from build123d import *

# Parameters (mm, degrees)
SKETCH4_W                               = 180
SKETCH4_H                               = 180
BOSS_EXTRUDE2_DEPTH                     = 10
SKETCH5_R                               = 70
BOSS_EXTRUDE3_DEPTH                     = 80
SKETCH7_R                               = 65
CUT_EXTRUDE1_DEPTH                      = 50
CBORE_FOR_M6_HEX_HEAD_BOLT2_D           = 6.6
CBORE_FOR_M6_HEX_HEAD_BOLT2_CBORE_D     = 14.55
CBORE_FOR_M6_HEX_HEAD_BOLT2_CBORE_DEPTH = 4.38
FILLET1_R                               = 10


with BuildPart() as part:
    # Sketch4 → Boss-Extrude2 (new body)
    with BuildSketch(Plane(origin=(0, 0, 0), x_dir=(1, 0, 0), z_dir=(0, 1, 0))):
        Rectangle(SKETCH4_W, SKETCH4_H)
    extrude(amount=BOSS_EXTRUDE2_DEPTH)

    # Sketch5 → Boss-Extrude3 (add)
    with BuildSketch(Plane(origin=(0, 10, 0), x_dir=(1, 0, 0), z_dir=(0, 1, 0))):
        with Locations(Location((0, 0, 0), (0, 0, 270))):
            Circle(SKETCH5_R)
    extrude(amount=BOSS_EXTRUDE3_DEPTH)

    # Sketch7 → Cut-Extrude1 (cut)
    with BuildSketch(Plane(origin=(0, 90, 0), x_dir=(1, 0, 0), z_dir=(0, 1, 0))):
        with Locations(Location((0, 0, 0), (0, 0, 270))):
            Circle(SKETCH7_R)
    extrude(amount=-CUT_EXTRUDE1_DEPTH, mode=Mode.SUBTRACT)

    # CBORE for M6 Hex Head Bolt2 (through all)
    with Locations(Plane(origin=(0, 10, 0), x_dir=(1, 0, 0), z_dir=(0, 1, 0))):
        with Locations((-75, 75), (75, 75), (75, -75), (-75, -75)):
            CounterBoreHole(CBORE_FOR_M6_HEX_HEAD_BOLT2_D / 2, CBORE_FOR_M6_HEX_HEAD_BOLT2_CBORE_D / 2, CBORE_FOR_M6_HEX_HEAD_BOLT2_CBORE_DEPTH)

    # Fillet1
    fillet1_edges = [part.edges().sort_by_distance(p)[0] for p in [
        (90, 5, 90),
        (-90, 5, 90),
        (-90, 5, -90),
        (90, 5, -90),
    ]]
    fillet(fillet1_edges, radius=FILLET1_R)


solid = part.part
Verification items for the finished model (mm, model axes). A direction names the side the tool comes from. Coordinates: 2 decimals unless noted, no trailing zeros. Order: outer loops, then holes, each group sorted by start corner. A loop starts at its lowest first (then second) coordinate and runs counter-clockwise, first axis right, second up. Notation, with made-up numbers: M 25,83.5 L 50,83.5 A12 cw 50,104.5 Z; hole C 78,4 d11. An arc over 180 degrees is marked long. Return JSON: item names as keys, results as strings.
1) Cross-section at D-D, the plane x = 0. Record the boundary of the cut face in (y, z), and give its area (3 significant figures).
Answer list:
{"outline": "M 0,-90 L 10,-90 L 10,-70 L 90,-70 L 90,-65 L 40,-65 L 40,65 L 90,65 L 90,70 L 10,70 L 10,90 L 0,90 Z", "area": "6,500 mm2"}
2) Cross-section at A-A, the plane z = 75. Record the boundary of the cut face in (x, y) (3 decimals), and give its area (3 significant figures).
Answer list:
{"outline": "M -90,0 L -78.3,0 L -78.3,5.62 L -82.275,5.62 L -82.275,10 L -90,10 Z; M -71.7,0 L 71.7,0 L 71.7,5.62 L 67.725,5.62 L 67.725,10 L -67.725,10 L -67.725,5.62 L -71.7,5.62 Z; M 78.3,0 L 90,0 L 90,10 L 82.275,10 L 82.275,5.62 L 78.3,5.62 Z", "area": "1,600 mm2"}
3) Thickness scan on L1, parallel to X at y = 8, z = 75 (3 decimals); L2, parallel to Z at x = 75, y = 3.85. Record the ranges inside material, lowest first. Write a range as [from, to].
Answer list:
{"L1": "[-90, -82.275], [-67.725, 67.725], [82.275, 90]", "L2": "[-90, -78.3], [-71.7, 71.7], [78.3, 90]"}
4) Access from +Z, -Z, +X, -X, +Y, -Y to the whole of each face (thin tool, end or side, straight path). Record for faces 5 (the flat face through (-90, 5, 1)), 6 (the cylindrical face through (-68.28, 7.84, -72.21)).
Answer list:
{"face 5": "+Z, -Z, -X, +Y, -Y", "face 6": "+Y"}
5) Cross-section at C-C, the plane z = 0. Record the boundary of the cut face in (x, y), and give its area (3 significant figures).
Answer list:
{"outline": "M -90,0 L 90,0 L 90,10 L 70,10 L 70,90 L 65,90 L 65,40 L -65,40 L -65,90 L -70,90 L -70,10 L -90,10 Z", "area": "6,500 mm2"}
6) Gauge pin test, flat ends, axial feed: pin 1 (6 mm diameter, centred on y = 69, z = -40.5, fed in from +X); pin 2 (6 mm diameter, centred on y = 78.5, z = -29.5, fed in from -X); pin 3 (6 mm diameter, centred on x = -7.5, y = 76.5, fed in from -Z). Record the tip position at first contact, or that the pin passes through.
Answer list:
{"pin 1": "x = 59.11", "pin 2": "x = -64.79", "pin 3": "z = -69.86"}
7) Cross-section at B-B, the plane x = -75. Record the boundary of the cut face in (y, z) (3 decimals).
Answer list:
{"outline": "M 0,-90 L 10,-90 L 10,-82.275 L 5.62,-82.275 L 5.62,-78.3 L 0,-78.3 Z; M 0,-71.7 L 5.62,-71.7 L 5.62,-67.725 L 10,-67.725 L 10,67.725 L 5.62,67.725 L 5.62,71.7 L 0,71.7 Z; M 0,78.3 L 5.62,78.3 L 5.62,82.275 L 10,82.275 L 10,90 L 0,90 Z"}
8) Release check for a two-part mould opening along Z. For faces 1 (the flat face through (-1, 5, -90)), 2 (the cylindrical face through (19.52, 65.35, 62)), 3 (the cylindrical face through (86.99, 5.07, 87.15)), 4 (the flat face through (-72, 5.62, 77)) record: +Z half, -Z half, draft (parallel to the pull), parting line (faces both ways), or undercut.
Answer list:
{"face 1": "-Z half", "face 2": "undercut", "face 3": "+Z half", "face 4": "undercut"}
